Could you check a few things on this model? Use its own coordinates, in mm. Coordinates: 2 decimals unless noted, no trailing zeros. Order: outer loops, then holes, each group sorted by start corner. A loop starts at its lowest first (then second) coordinate and runs counter-clockwise, first axis right, second up. Notation, with made-up numbers: (30, 73) - (41, 73) arc R27 cw to (41, 103) - close; hole circle Ø5 at (62.5, 23.5). An arc over 180 degrees is marked (long way). One line per item, written item: value.
from build123d import *

# Parameters (mm, degrees)
ESQUISSE1_W             = 10
ESQUISSE1_H             = 50
BOSS_EXTRU_1_DEPTH      = 10
ESQUISSE2_R             = 2
ENL_V_MAT_EXTRU_1_DEPTH = 10
CONG_1_R                = 5


with BuildPart() as part:
    # Esquisse1 → Boss.-Extru.1 (new body)
    with BuildSketch(Plane.XY):
        with Locations((5, 25)):
            Rectangle(ESQUISSE1_W, ESQUISSE1_H)
    extrude(amount=BOSS_EXTRU_1_DEPTH)

    # Esquisse2 → Enlèv. mat.-Extru.1 (cut)
    with BuildSketch(Plane.XY.offset(10)):
        with Locations((5, 45)):
            Circle(ESQUISSE2_R)
        with Locations((5, 5)):
            Circle(ESQUISSE2_R)
    extrude(amount=-ENL_V_MAT_EXTRU_1_DEPTH, mode=Mode.SUBTRACT)

    # Congé1
    cong_1_edges = [part.edges().sort_by_distance(p)[0] for p in [
        (10, 50, 5),
        (0, 50, 5),
        (10, 0, 5),
        (0, 0, 5),
    ]]
    fillet(cong_1_edges, radius=CONG_1_R - 0.0001)  # a hair under: the kernel refuses the full size


solid = part.part
Item 1: I want a section at C-C on x = 2.5. Please give me the cut outline in (y, z), then the cut area to 3 significant figures.
Conclusion:
outline: (0.67, 0) - (49.33, 0) - (49.33, 10) - (0.67, 10) - close
area: 487 mm²
Item 2: If I drill on probe 1 along Y at (x, z) = (5, 5.25); probe 2 along Y at (x, z) = (5.75, 7.75); probe 3 along Y at (x, z) = (2, 3.25), over which ranges is the centre line in solid material (lowest first)?
Conclusion:
probe 1: 0 to 3, 7 to 43, 47 to 50
probe 2: 0.06 to 3.15, 6.85 to 43.15, 46.85 to 49.94
probe 3: 1 to 49
Item 3: I want a section at D-D on x = 8.5. Please give me the cut outline in (y, z).
Conclusion:
outline: (1.43, 0) - (48.57, 0) - (48.57, 10) - (1.43, 10) - close
Item 4: Thinking about a two-plate mould opening in X: for faces 1 (the face through (5, 25, 10)), 2 (the face through (8, 49, 5)), 3 (the face through (5, 43, 5)), 4 (the face through (3, 5, 5)), which applies, pulls with the +X half, pulls with the -X half, needs draft (parallel to the pull), parting line crosses it, or undercut?
Conclusion:
face 1: needs draft
face 2: pulls with the +X half
face 3: undercut
face 4: undercut
Item 5: I'm going to push flat-ended pins straight in: pin 1 Ø3.5 at (x, y) = (5, 45) entering from +Z; pin 2 Ø5 at (x, y) = (3.5, 40.5) entering from -Z; pin 3 Ø1 at (x, z) = (6, 6) entering from -Y; pin 4 Ø1.5 at (x, z) = (4, 4) entering from +Y. Where does each tip first touch, or does it pass through?
Conclusion:
pin 1: through
pin 2: z = 0
pin 3: y = 0.03
pin 4: y = 49.99
Item 6: I want a section at B-B on x = 6.25. Please give me the cut outline in (y, z).
Conclusion:
outline: (0.16, 0) - (3.44, 0) - (3.44, 10) - (0.16, 10) - close; (6.56, 0) - (43.44, 0) - (43.44, 10) - (6.56, 10) - close; (46.56, 0) - (49.84, 0) - (49.84, 10) - (46.56, 10) - close
Item 7: I want a section at A-A on z = 2.5. Give the number of separate pieces and of enclosed holes in the cut face, then the cut area to 3 significant figures.
Conclusion:
separate pieces: 1
enclosed holes: 2
area: 453 mm²
